The listing builds one solid part. Answer for the finished solid, in the listing's coordinates (mm). Round coordinates to 2 decimals unless told otherwise and drop trailing zeros. Order: outer loops, then holes, each group sorted by start corner. A loop starts at its lowest first (then second) coordinate and runs counter-clockwise, first axis right, second up. Notation, with made-up numbers: M 76,63.25 L 127,63.25 A26 ccw 127,88.25 Z; hole C 81.25,-28.5 d8. An arc over 180 degrees is marked long. Write item = value, one per line. Start each with the question number.
(1) Straight lines are drawn through the part: probe 1 along Y at (x, z) = (9, 4.25); probe 2 along X at (y, z) = (53.5, 5.75); probe 3 along Y at (x, z) = (78, 2). For each, find the intervals that lie inside material, in ascending order. Write a range as from..to.
(2) A cutting plane is placed at A-A, the plane x = 162. Determine the outline of the cut face in (y, z), and give its area (3 significant figures).
(3) A cutting plane is placed at D-D, the plane y = 28.5. Determine the outline of the cut face in (x, z), and give its area (3 significant figures).
(4) A cutting plane is placed at B-B, the plane z = 6. Count the separate pieces of the cut face and the enclosed holes in it, and give its area (3 significant figures).
(5) A cutting plane is placed at C-C, the plane x = 18. Determine the outline of the cut face in (y, z).
(6) Each of these flat-tipped pins is pushed along its axis until it touches: pin 1 (3 mm diameter, centred on x = 78, y = 10, fed in from +Z); pin 2 (6.5 mm diameter, centred on x = 318, y = 10, fed in from -Z); pin 3 (1 mm diameter, centred on x = 65.5, z = 5, fed in from +Y). Where does it stop, or does it pass through?
Autodesk Inventor part; units mm, degrees
ref_plane "YZ Plane" through (0, 0, 0) normal (1, 0, 0) x (0, 1, 0)
ref_plane "XZ Plane" through (0, 0, 0) normal (0, 1, 0) x (-1, 0, 0)
ref_plane "XY Plane" through (0, 0, 0) normal (0, 0, 1) x (1, 0, 0)
sketch "Sketch1" plane through (0, 0, 0) normal (0, 0, 1) x (1, 0, 0)
  line L0 (0, 0) -> (18.2608, 0)
  line L1 (42, 25) -> (42, 60)
  line L2 (42, 60) -> (0, 60)
  line L3 (0, 60) -> (0, 0)
  line L4 (47, 20) -> (330, 20)
  line L5 (330, 20) -> (330, 0)
  line L6 (330, 0) -> (18.2608, 0)
  circle A0 centre (9, 54) radius 2.05
  circle A1 centre (33, 54) radius 2.05
  circle A2 centre (33, 38) radius 2.05
  circle A3 centre (9, 38) radius 2.05
  line L7 (42, 25) -> (47, 20)
  point P0 (42, 20)
  dimension "d0" = 330
  dimension "d1" = 60
  dimension "d2" = 42
  dimension "d3" = 40
  dimension "d4" = 4.1
  dimension "d5" = 24
  dimension "d6" = 16
  dimension "d7" = 6
  dimension "d8" = 9
  dimension "d9" = 5
  dimension "d10" = 5
extrude "Extrusion1" add sketch "Sketch1" along normal blind 10
sketch "Sketch2" plane through (0, 0, 10) normal (0, 0, 1) x (1, 0, 0)
  line L0 (330, 20) -> (330, 0)
  line L1 (47, 20) -> (330, 20)
  circle A0 centre (318, 10) radius 2
  circle A1 centre (306, 10) radius 6
  line L2 (336.598, 10) -> (-63.669, 10) construction
  circle A2 centre (294, 10) radius 2
  circle A3 centre (282, 10) radius 6
  line L3 (312.598, 10) -> (-87.669, 10) construction
  circle A4 centre (270, 10) radius 2
  circle A5 centre (258, 10) radius 6
  line L4 (288.598, 10) -> (-111.669, 10) construction
  circle A6 centre (246, 10) radius 2
  circle A7 centre (234, 10) radius 6
  line L5 (264.598, 10) -> (-135.669, 10) construction
  circle A8 centre (222, 10) radius 2
  circle A9 centre (210, 10) radius 6
  line L6 (240.598, 10) -> (-159.669, 10) construction
  circle A10 centre (198, 10) radius 2
  circle A11 centre (186, 10) radius 6
  line L7 (216.598, 10) -> (-183.669, 10) construction
  circle A12 centre (174, 10) radius 2
  circle A13 centre (162, 10) radius 6
  line L8 (192.598, 10) -> (-207.669, 10) construction
  circle A14 centre (150, 10) radius 2
  circle A15 centre (138, 10) radius 6
  line L9 (168.598, 10) -> (-231.669, 10) construction
  circle A16 centre (126, 10) radius 2
  circle A17 centre (114, 10) radius 6
  line L10 (144.598, 10) -> (-255.669, 10) construction
  circle A18 centre (102, 10) radius 2
  circle A19 centre (90, 10) radius 6
  line L11 (120.598, 10) -> (-279.669, 10) construction
  circle A20 centre (78, 10) radius 2
  circle A21 centre (66, 10) radius 6
  line L12 (96.598, 10) -> (-303.669, 10) construction
  circle A22 centre (54, 10) radius 2
  circle A23 centre (42, 10) radius 6
  line L13 (72.598, 10) -> (-327.669, 10) construction
  circle A24 centre (30, 10) radius 2
  circle A25 centre (18, 10) radius 6
  line L14 (48.598, 10) -> (-351.669, 10) construction
  dimension "d13" = 10
  dimension "d14" = 12
  dimension "d15" = 4
  dimension "d16" = 12
  dimension "d17" = 12
  dimension "d20" = 24
extrude "Extrusion2" cut sketch "Sketch2" against normal through all
equation "\"d8\" = -0.5 * d5 + 0.5 * d2"
properties part number "Set Square"
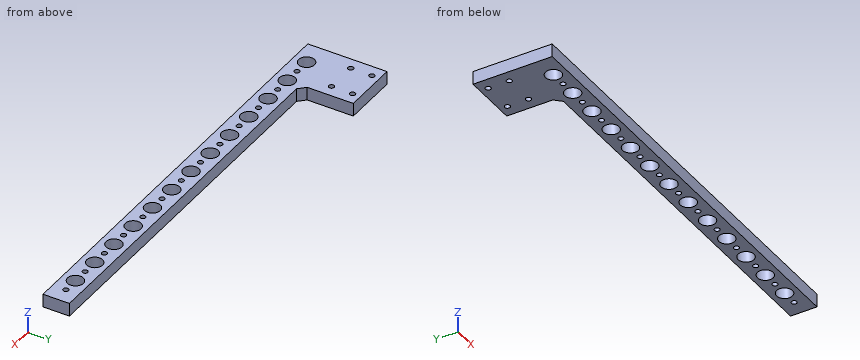
Reported:
q1.probe_1 = 0..35.95, 40.05..51.95, 56.05..60
q1.probe_2 = 0..7.01, 10.99..31.01, 34.99..42
q1.probe_3 = 0..8, 12..20
q2.outline = M 0,0 L 4,0 L 4,10 L 0,10 Z; M 16,0 L 20,0 L 20,10 L 16,10 Z
q2.area = 80.0 mm²
q3.outline = M 0,0 L 42,0 L 42,10 L 0,10 Z
q3.area = 420 mm²
q4.separate_pieces = 1
q4.enclosed_holes = 30
q4.area = 6,610 mm²
q5.outline = M 0,0 L 4,0 L 4,10 L 0,10 Z; M 16,0 L 60,0 L 60,10 L 16,10 Z
q6.pin_1 = through
q6.pin_2 = 0
q6.pin_3 = 20
